```python
from build123d import *

# Parameters (mm, degrees)
SKETCH1_R                 = 4
BOSS_EXTRUDE1_DEPTH       = 22
BOSS_EXTRUDE2_DEPTH       = 24
BOSS_EXTRUDE2_DEPTH_BACK  = 2
SKETCH1_3_R               = 4
SKETCH1_3_R_2             = 3
CUT_EXTRUDE1_DEPTH        = 18
BOSS_EXTRUDE3_DEPTH       = 3
SKETCH3_W                 = 1
SKETCH3_H                 = 1
CUT_EXTRUDE2_DEPTH        = 2
BOSS_EXTRUDE7_START       = -1
BOSS_EXTRUDE7_DEPTH       = 1
BOSS_EXTRUDE8_DEPTH       = 5
CUT_EXTRUDE8_REACH        = 33.953
SKETCH8_R                 = 1
FILLET1_R                 = 0.5
F_4_0MM_DOWEL_HOLE1_D     = 4
F_4_0MM_DOWEL_HOLE1_DEPTH = 5.798278762
F_4_0MM_DOWEL_HOLE1_TIP   = 1.201721238
F_3_0MM_DOWEL_HOLE1_D     = 3
F_3_0MM_DOWEL_HOLE1_DEPTH = 6.098709071
F_3_0MM_DOWEL_HOLE1_TIP   = 0.901290929


with BuildPart() as part:
    # Sketch1 → Boss-Extrude1 (new body)
    with BuildSketch(Plane(origin=(0, 0, 0), x_dir=(1, 0, 0), z_dir=(0, 1, 0))):
        with BuildLine():
            Line((-5.656854249, 2), (-8.535898385, 2))
            ThreePointArc((-8.535898385, 2), (-16, 0), (-8.535898385, -2))
            Line((-8.535898385, -2), (-5.656854249, -2))
            ThreePointArc((-5.656854249, -2), (6, 0), (-5.656854249, 2))
        make_face()
        with Locations(Location((0, 0, 0), (0, 0, 270))):
            Circle(SKETCH1_R, mode=Mode.SUBTRACT)
    extrude(amount=BOSS_EXTRUDE1_DEPTH)

    # Sketch1<3> → Boss-Extrude2 (add, two sides: drawn at the far end of the back side and taken through both)
    with BuildSketch(Plane(origin=(0, 0, 0), x_dir=(1, 0, 0), z_dir=(0, 1, 0)).offset(-BOSS_EXTRUDE2_DEPTH_BACK)):
        with Locations(Location((0, 0, 0), (0, 0, 270))):
            Circle(SKETCH1_3_R)
        with Locations(Location((0, 0, 0), (0, 0, 270))):
            Circle(SKETCH1_3_R_2, mode=Mode.SUBTRACT)
    extrude(amount=BOSS_EXTRUDE2_DEPTH + BOSS_EXTRUDE2_DEPTH_BACK)

    # Sketch2 → Cut-Extrude1 (cut)
    with BuildSketch(Plane(origin=(0, 4, 0), x_dir=(1, 0, 0), z_dir=(0, 1, 0))):
        with BuildLine():
            ThreePointArc((5.656854249, 2), (5.368939451, 2.678523692), (5, 3.31662479))
            Line((5, 3.31662479), (5, 0))
            Line((5, 0), (6, 0))
            ThreePointArc((6, 0), (5.913591358, 1.014611872), (5.656854249, 2))
        make_face()
        with BuildLine():
            Line((6, 0), (5, 0))
            Line((5, 0), (5, -3.31662479))
            ThreePointArc((5, -3.31662479), (5.368939451, -2.678523692), (5.656854249, -2))
            ThreePointArc((5.656854249, -2), (5.913591358, -1.014611872), (6, 0))
        make_face()
    extrude(amount=CUT_EXTRUDE1_DEPTH, mode=Mode.SUBTRACT)

    # Sketch2<3> → Boss-Extrude3 (add)
    with BuildSketch(Plane(origin=(0, 4, 0), x_dir=(1, 0, 0), z_dir=(0, 1, 0))):
        with BuildLine():
            Line((5, 3.31662479), (5, -3.31662479))
            ThreePointArc((5, -3.31662479), (5.368939451, -2.678523692), (5.656854249, -2))
            Line((5.656854249, -2), (7, -2))
            Line((7, -2), (7, -1))
            Line((7, -1), (8, -1))
            Line((8, -1), (8, -2))
            Line((8, -2), (9, -2))
            Line((9, -2), (9, 2))
            Line((9, 2), (8, 2))
            Line((8, 2), (8, 1))
            Line((8, 1), (7, 1))
            Line((7, 1), (7, 2))
            Line((7, 2), (5.656854249, 2))
            ThreePointArc((5.656854249, 2), (5.368939451, 2.678523692), (5, 3.31662479))
        make_face()
    extrude(amount=BOSS_EXTRUDE3_DEPTH)

    # Sketch3 → Cut-Extrude2 (cut)
    with BuildSketch(Plane.XY.offset(1)):
        with Locations((7.5, 4.5)):
            Rectangle(SKETCH3_W, SKETCH3_H)
    extrude(amount=-CUT_EXTRUDE2_DEPTH, mode=Mode.SUBTRACT)

    # Sketch6 → Boss-Extrude7 (add)
    with BuildSketch(Plane(origin=(0, 22, 0), x_dir=(1, 0, 0), z_dir=(0, 1, 0)).offset(BOSS_EXTRUDE7_START)):
        Polygon((-9.856725658, -4.596266659), (-6.232597162, -2.906307787), (-6.655215424, -2), (-10.27934392, -3.689958872), align=None)
        Polygon((-6.232597162, -2.906307787), (-5.412549479, -2.523913272), (-5.83516774, -1.617605485), (-6.655215424, -2), align=None)
        with BuildLine():
            Line((-10.27934392, -3.689958872), (-6.655215424, -2))
            Line((-6.655215424, -2), (-8.535898385, -2))
            ThreePointArc((-8.535898385, -2), (-9.29763917, -2.949109347), (-10.309526953, -3.625231148))
            Line((-10.309526953, -3.625231148), (-10.27934392, -3.689958872))
        make_face()
    extrude(amount=BOSS_EXTRUDE7_DEPTH)

    # Sketch7 → Boss-Extrude8 (add)
    with BuildSketch(Plane(origin=(0, 22, 0), x_dir=(1, 0, 0), z_dir=(0, 1, 0))):
        Polygon((-10.27934392, -3.689958872), (-6.654112772, -1.999485825), (-6.23149451, -2.905793612), (-9.856725658, -4.596266659), align=None)
    extrude(amount=BOSS_EXTRUDE8_DEPTH)

    # Sketch8 → Cut-Extrude8 (cut, up to next)
    with BuildSketch(Plane(origin=(0, 0, 0), x_dir=(0.9063077870366509, 0, -0.42261826174069733), z_dir=(0.42261826174069733, 0, 0.9063077870366509)), mode=Mode.PRIVATE) as cut_extrude8_sk1:
        with BuildLine():
            ThreePointArc((-10.875693444, 25), (-10.289907007, 26.414213562), (-8.875693444, 27))
            Line((-8.875693444, 27), (-10.875693444, 27))
            Line((-10.875693444, 27), (-10.875693444, 25))
        make_face()
    cut_extrude8_tool1 = extrude(cut_extrude8_sk1.sketch, amount=-CUT_EXTRUDE8_REACH, mode=Mode.PRIVATE) & part.part
    # Sketch8 → Cut-Extrude8 (cut, up to next)
    with BuildSketch(Plane(origin=(0, 0, 0), x_dir=(0.9063077870366509, 0, -0.42261826174069733), z_dir=(0.42261826174069733, 0, 0.9063077870366509)), mode=Mode.PRIVATE) as cut_extrude8_sk2:
        with BuildLine():
            ThreePointArc((-8.875693444, 27), (-7.461479882, 26.414213562), (-6.875693444, 25))
            Line((-6.875693444, 25), (-6.875693444, 27))
            Line((-6.875693444, 27), (-8.875693444, 27))
        make_face()
    cut_extrude8_tool2 = extrude(cut_extrude8_sk2.sketch, amount=-CUT_EXTRUDE8_REACH, mode=Mode.PRIVATE) & part.part
    # Sketch8 → Cut-Extrude8 (cut, up to next)
    with BuildSketch(Plane(origin=(0, 0, 0), x_dir=(0.9063077870366509, 0, -0.42261826174069733), z_dir=(0.42261826174069733, 0, 0.9063077870366509)), mode=Mode.PRIVATE) as cut_extrude8_sk3:
        with Locations((-8.875693444, 25)):
            Circle(SKETCH8_R)
    cut_extrude8_tool3 = extrude(cut_extrude8_sk3.sketch, amount=-CUT_EXTRUDE8_REACH, mode=Mode.PRIVATE) & part.part
    add(cut_extrude8_tool1.solids().sort_by_distance((-9.451845, 26.553264, 4.407468))[0], mode=Mode.SUBTRACT)
    add(cut_extrude8_tool2.solids().sort_by_distance((-6.636375, 26.553264, 3.094592))[0], mode=Mode.SUBTRACT)
    add(cut_extrude8_tool3.solids().sort_by_distance((-8.04411, 25, 3.75103))[0], mode=Mode.SUBTRACT)

    # Fillet1
    # the kernel refuses this fillet: 0.5 mm, written as the material it adds along each edge
    with BuildSketch(Plane(origin=(-5.437846722, 22, 2.53570957), x_dir=(0.4571889357830061, 0, 0.8893695952738672), z_dir=(0, -1, 0))) as fillet1_piece_1:
        with BuildLine():
            CenterArc((0.481125753, 0.499629492), FILLET1_R, 182.205862892, 85.588274215)
            Line((-0.018503738, 0.480384461), (0, 0))
            ThreePointArc((0, 0), (0.230940361, 0.004446102), (0.461880723, 0))
        make_face()
    extrude(amount=1)
    with BuildSketch(Plane(origin=(-10.309526953, 21, 3.625231148), x_dir=(-0.9284189548945215, 0, 0.3715349838071298), z_dir=(0, 1, 0))) as fillet1_piece_2:
        with BuildLine():
            CenterArc((0.472954925, 0.499225399), FILLET1_R, 183.189685104, 83.620629792)
            Line((-0.026270474, 0.471404521), (0, 0))
            ThreePointArc((0, 0), (0.222567024, 0.00619681), (0.445134047, 0))
        make_face()
    extrude(amount=1)

    # Ø4.0mm Dowel Hole1
    with Locations(Plane(origin=(0, 0, 0), x_dir=(-1, 0, 0), z_dir=(0, -1, 0))):
        with Locations((12, 0)):
            Hole(F_4_0MM_DOWEL_HOLE1_D / 2, depth=F_4_0MM_DOWEL_HOLE1_DEPTH)
            with Locations((0, 0, -(F_4_0MM_DOWEL_HOLE1_DEPTH + F_4_0MM_DOWEL_HOLE1_TIP / 2))):  # 118° drill point
                Cone(0, F_4_0MM_DOWEL_HOLE1_D / 2, F_4_0MM_DOWEL_HOLE1_TIP, mode=Mode.SUBTRACT)

    # Ø3.0mm Dowel Hole1
    with Locations(Plane(origin=(0, 22, 0), x_dir=(1, 0, 0), z_dir=(0, 1, 0))):
        with Locations((-12, 0)):
            Hole(F_3_0MM_DOWEL_HOLE1_D / 2, depth=F_3_0MM_DOWEL_HOLE1_DEPTH)
            with Locations((0, 0, -(F_3_0MM_DOWEL_HOLE1_DEPTH + F_3_0MM_DOWEL_HOLE1_TIP / 2))):  # 118° drill point
                Cone(0, F_3_0MM_DOWEL_HOLE1_D / 2, F_3_0MM_DOWEL_HOLE1_TIP, mode=Mode.SUBTRACT)


solid = part.part
```
CAD build for the part. Positions are in the model's coordinates, mm. A direction names the side the tool comes from. Give positions to 0.01 mm unless a question says otherwise; leave off trailing zeros. Order: outer loops, then holes, each group sorted by start corner. A loop starts at its lowest first (then second) coordinate and runs counter-clockwise, first axis right, second up.
(1) Mould opens along X. For faces 6 (the flat face through (8.5, 5.5, 2)), 7 (the cylindrical face through (-16, 11, 0)), 8 (the flat face through (-10.065, 22.972, 4.149)) say: released by +X, released by -X, zero draft, split by the parting line, or undercut.
(2) Drill centre lines: L1, parallel to Z at x = -12, y = 19.25; L2, parallel to X at y = 18, z = -2.5; L3, parallel to Z at x = -12, y = 1.3. Where is each one in solid material? Low to high.
(3) Flat gauge pins, fed straight in: pin 1 (1.1 mm diameter, centred on x = 7.5, y = 5.5, fed in from -Z); pin 2 (4.5 mm diameter, centred on x = 7.5, z = -1, fed in from +Y); pin 3 (5.5 mm diameter, centred on y = 13.5, z = 0.5, fed in from +X); pin 4 (10 mm diameter, centred on x = -3, y = 22, fed in from +Z). Where does each tip first touch, or does it go through?
(4) Tool access for faces 1 (the flat face through (-6.446, 23.479, 2.446)), 2 (the flat face through (6, 5, 2)), 3 (the cylindrical face through (-3.905, 22.986, -0.867)), 4 (the flat face through (5, 14, 0)), 5 (the flat face through (8.5, 4, 0)): list every direction of +Z, -Z, +X, -X, +Y, -Y with a clear straight run to the whole face (end or side of a thin tool).
(5) Saw through at A-A, the plane x = 0. Give the cut face in (y, z).
(6) Saw through at C-C, the plane y = 14.5. Give the cut face in (x, z).
(7) Saw through at B-B, the plane y = 2.5. Give the cut face in (x, z), then the cut area to 3 significant figures.
Results found:
1. face 6: zero draft
1. face 7: undercut
1. face 8: released by -X
2. L1: z = -4 to -1.5, 1.5 to 4
2. L2: x = -15.12 to -8.88, -5.45 to -1.66, 1.66 to 5
2. L3: z = -4 to -2, 2 to 4
3. pin 1: stops at z = -2
3. pin 2: stops at y = 7
3. pin 3: stops at x = 5
3. pin 4: stops at z = 6
4. face 1: -Z, +Y
4. face 2: +Z, +X, +Y, -Y
4. face 3: +Y
4. face 4: +Z, -Z, +X, +Y
4. face 5: +Z, -Z, +X, -Y
5. outline: (-2, -4) - (0, -4) - (0, -6) - (22, -6) - (22, -4) - (24, -4) - (24, -3) - (-2, -3) - close; (-2, 3) - (24, 3) - (24, 4) - (22, 4) - (22, 6) - (0, 6) - (0, 4) - (-2, 4) - close
6. outline: (-8.54, -2) - (-5.66, -2) arc R6 ccw to (5, -3.32) - (5, 3.32) arc R6 ccw to (-5.66, 2) - (-8.54, 2) arc R4 ccw (long way) to start; hole circle Ø6 at (0, 0)
7. outline: (-8.54, -2) - (-5.66, -2) arc R6 ccw (long way) to (-5.66, 2) - (-8.54, 2) arc R4 ccw (long way) to start; hole circle Ø4 at (-12, 0); hole circle Ø6 at (0, 0)
7. area: 132 mm2
